Read the model definition and answer for the solid it produces. Units are mm, in the model's axes. A direction names the side the tool comes from. Coordinates: 2 decimals unless noted, no trailing zeros. Loops run counter-clockwise (first coordinate to the right, second up) from the corner with the lowest first, then second, coordinate; pieces in that order, holes last. Notation, with made-up numbers: (56, 28.25) - (104, 28.25) arc R5 cw to (104, 37.25) - close; hole circle Ø9 at (-30.5, 76). An arc over 180 degrees is marked (long way). One line per question, with ' | ' between items. Start each with the question number.
```python
from build123d import *

# Parameters (mm, degrees)
F0_W     = 76.2
F0_H     = 76.2
F1_DEPTH = 3.175
F3_DEPTH = 76.2
F4_W     = 19.098544
F4_H     = 24.549261
F5_DEPTH = 4


with BuildPart() as f1:
    # F0 (on Top) → F1 (new body)
    with BuildSketch(Plane.XY):
        with Locations((-12.826032, -9.711786)):
            Rectangle(F0_W, F0_H)
    extrude(amount=F1_DEPTH)

    # F2 (on face) → F3 (join)
    with BuildSketch(Plane(origin=(-50.926032, 0, 0), x_dir=(0, -1, 0), z_dir=(-1, 0, 0))):
        Polygon((1.052486, 74.779578), (-0.483229, 70.560237), (24.38552, 17.229033), (27.888745, 17.229033), (26.499598, 20.208069), align=None)
        Polygon((45.305423, 35.98803), (26.499598, 20.208069), (27.888745, 17.229033), (47.346274, 33.555839), align=None)
        Polygon((-2.326279, 74.779578), (-28.388214, 3.175), (-25.009449, 3.175), (-0.483229, 70.560237), (1.052486, 74.779578), align=None)
    extrude(amount=-F3_DEPTH)

    # F4 (on face) → F5 (cut)
    with BuildSketch(Plane(origin=(0, -0.998464, -1.189923), x_dir=(1, 0, 0), z_dir=(0, 0.642788, 0.766044))):
        with Locations((-12.696923, -45.563997)):
            Rectangle(F4_W, F4_H)
    extrude(amount=-F5_DEPTH, mode=Mode.SUBTRACT)


solid = f1.part
```
1) Find the intervals of material crossed by line 1 along Y through (x, z) = (-29.5, 33); line 2 along Y through (x, z) = (5.5, 30); line 3 along Z through (x, y) = (7, -20) (1 decimal), in increasing order. Write a range as from..to.
2) The part is cut by section C-C on z = 32.5. Write down the section's boundary in (x, y).
3) The part is cut by section A-A on x = 0.5. Write down the section's boundary in (y, z) (3 decimals), and give its area (3 significant figures).
4) The part is cut by section B-B on y = -39. Write down the section's boundary in (x, z) (3 decimals), and give its area (3 significant figures).
5) Which of the six approach directions +Z, -Z, +X, -X, +Y, -Y give full straight-line access (tool end or side, diameter ignored) to faces 1 (the flat face through (-3.148, -37, 27)), 2 (the flat face through (-13, -26, 17.229)), 3 (the flat face through (10.864, -36.034, 28.209)), 4 (the flat face through (-13, 28.388, 2)), 5 (the flat face through (-13.359, -11.777, 44.268))?
6) The mould has two halves that part along Y. Classify faces 6 (the flat face through (-22.246, -37, 27)), 7 (the flat face through (-36.787, -36.034, 28.209)), 8 (the flat face through (-12.831, -27.506, 19.009)): released by +Y, released by -Y, zero draft, split by the parting line, or undercut.
7) The part is cut by section D-D on y = -16.5. Write down the section's boundary in (x, z) (3 decimals).
8) Given pin 1 Ø10 at (x, z) = (-22, 32) entering from +Y; pin 2 Ø1 at (x, z) = (-14.5, 65) entering from -Y; pin 3 Ø8 at (x, z) = (10, 45) entering from +Y, each flat-ended and moving along its own axis, determine where each tip first touches the part or whether it passes through.
Answer below:
1) line 1: -46.68..-41.74, -20.53..-17.03, 14.15..17.53 | line 2: -43.11..-38.17, -21.93..-18.43, 15.25..18.62 | line 3: 0..3.2, 26.6..34.1
2) outline: (-50.93, -46.09) - (-22.25, -46.09) - (-22.25, -41.15) - (-50.93, -41.15) - close; (-50.93, -20.77) - (25.27, -20.77) - (25.27, -17.26) - (-50.93, -17.26) - close; (-50.93, 14.34) - (25.27, 14.34) - (25.27, 17.71) - (-50.93, 17.71) - close; (-3.15, -46.09) - (25.27, -46.09) - (25.27, -41.15) - (-3.15, -41.15) - close
3) outline: (-47.812, 0) - (28.388, 0) - (28.388, 3.175) - (2.326, 74.78) - (-1.052, 74.78) - (-26.5, 20.208) - (-45.305, 35.988) - (-47.346, 33.556) - (-27.889, 17.229) - (-24.386, 17.229) - (0.483, 70.56) - (25.009, 3.175) - (-47.812, 3.175) - close | area: 757 mm2
4) outline: (-50.926, 0) - (25.274, 0) - (25.274, 3.175) - (-50.926, 3.175) - close; (-50.926, 26.552) - (-22.246, 26.552) - (-22.246, 30.697) - (-50.926, 30.697) - close; (-3.148, 26.552) - (25.274, 26.552) - (25.274, 30.697) - (-3.148, 30.697) - close | area: 479 mm2
5) face 1: +Z, -Y | face 2: +X, -X, -Y | face 3: +Z, +X, -X | face 4: +Z, -Z, +X, -X, +Y | face 5: +X, -X
6) face 6: zero draft | face 7: undercut | face 8: released by -Y
7) outline: (-50.926, 0) - (25.274, 0) - (25.274, 3.175) - (-50.926, 3.175) - close; (-50.926, 34.14) - (25.274, 34.14) - (25.274, 41.652) - (-50.926, 41.652) - close
8) pin 1: y = 19.72 | pin 2: y = -5.85 | pin 3: y = 14.62
